from build123d import *

# Parameters (mm, degrees)
F1_DEPTH     = 6.35
F2_T1_DEPTH  = 59.8574546933
F2_T3_DEPTH  = 28.1503971994
F2_T6_ANGLE  = 90
F2_T8_ANGLE  = 90
F2_T10_ANGLE = 90
F2_T12_ANGLE = 90


# Not quite as in the source:
# - a fillet or chamfer that OpenCascade refuses, or shapes differently, is made with other operations: its cross-section is extruded or revolved along the edge and cut away or added


with BuildPart() as f1:
    # F0 (on Top) → F1 (new body)
    with BuildSketch(Plane.XY):
        with BuildLine():
            Line((20.4174276441, 0), (-20.4329695553, 0))
            Line((-20.4329695553, 0), (-20.4329695553, -47.1574546933))
            ThreePointArc((-20.4329695553, -47.1574546933), (-18.5730976158, -51.6475827539), (-14.0829695553, -53.5074546933))
            Line((-14.0829695553, -53.5074546933), (14.0674276441, -53.5074546933))
            ThreePointArc((14.0674276441, -53.5074546933), (18.5575557047, -51.6475827539), (20.4174276441, -47.1574546933))
            Line((20.4174276441, -47.1574546933), (20.4174276441, 0))
        make_face()
    extrude(amount=F1_DEPTH)

    # F2: fillet of radius 5.08 on 10 edges, made by hand

    # F2_s2 → F2_t1 (cut)
    with BuildSketch(Plane.XZ.offset(-12.7)):
        with BuildLine():
            ThreePointArc((20.4174276441, 1.27), (18.9295300926, 4.8621024484), (15.3374276441, 6.35))
            Line((15.3374276441, 6.35), (20.4174276441, 6.35))
            Line((20.4174276441, 6.35), (20.4174276441, 1.27))
        make_face()
        with BuildLine():
            ThreePointArc((20.4174276441, 5.08), (18.9295300926, 1.4878975516), (15.3374276441, 0))
            Line((15.3374276441, 0), (20.4174276441, 0))
            Line((20.4174276441, 0), (20.4174276441, 5.08))
        make_face()
        with BuildLine():
            ThreePointArc((-20.4329695553, 1.27), (-18.9450720037, 4.8621024484), (-15.3529695553, 6.35))
            Line((-15.3529695553, 6.35), (-20.4329695553, 6.35))
            Line((-20.4329695553, 6.35), (-20.4329695553, 1.27))
        make_face()
        with BuildLine():
            ThreePointArc((-20.4329695553, 5.08), (-18.9450720037, 1.4878975516), (-15.3529695553, 0))
            Line((-15.3529695553, 0), (-20.4329695553, 0))
            Line((-20.4329695553, 0), (-20.4329695553, 5.08))
        make_face()
    extrude(amount=F2_T1_DEPTH, mode=Mode.SUBTRACT)

    # F2_s4 → F2_t3 (cut)
    with BuildSketch(Plane.YZ.offset(-14.0829695553)):
        with BuildLine():
            ThreePointArc((-53.5074546933, 5.08), (-52.0195571417, 1.4878975516), (-48.4274546933, 0))
            Line((-48.4274546933, 0), (-53.5074546933, 0))
            Line((-53.5074546933, 0), (-53.5074546933, 5.08))
        make_face()
        with BuildLine():
            ThreePointArc((-53.5074546933, 1.27), (-52.0195571417, 4.8621024484), (-48.4274546933, 6.35))
            Line((-48.4274546933, 6.35), (-53.5074546933, 6.35))
            Line((-53.5074546933, 6.35), (-53.5074546933, 1.27))
        make_face()
    extrude(amount=F2_T3_DEPTH, mode=Mode.SUBTRACT)

    # F2_s5 → F2_t6 (revolve, cut)
    with BuildSketch(Plane.YZ.offset(14.0674276441)):
        with BuildLine():
            ThreePointArc((-53.5074546933, 1.27), (-52.0195571417, 4.8621024484), (-48.4274546933, 6.35))
            Line((-48.4274546933, 6.35), (-53.5074546933, 6.35))
            Line((-53.5074546933, 6.35), (-53.5074546933, 1.27))
        make_face()
    revolve(axis=Axis((14.0674276441, -47.1574546933, 6.35), (0, 0, 1)), revolution_arc=F2_T6_ANGLE, mode=Mode.SUBTRACT)

    # F2_s7 → F2_t8 (revolve, cut)
    with BuildSketch(Plane.YZ.offset(14.0674276441)):
        with BuildLine():
            ThreePointArc((-53.5074546933, 5.08), (-52.0195571417, 1.4878975516), (-48.4274546933, 0))
            Line((-48.4274546933, 0), (-53.5074546933, 0))
            Line((-53.5074546933, 0), (-53.5074546933, 5.08))
        make_face()
    revolve(axis=Axis((14.0674276441, -47.1574546933, 0), (0, 0, 1)), revolution_arc=F2_T8_ANGLE, mode=Mode.SUBTRACT)

    # F2_s9 → F2_t10 (revolve, cut)
    with BuildSketch(Plane.XZ.offset(47.1574546933)):
        with BuildLine():
            ThreePointArc((-20.4329695553, 1.27), (-18.9450720037, 4.8621024484), (-15.3529695553, 6.35))
            Line((-15.3529695553, 6.35), (-20.4329695553, 6.35))
            Line((-20.4329695553, 6.35), (-20.4329695553, 1.27))
        make_face()
    revolve(axis=Axis((-14.0829695553, -47.1574546933, 6.35), (0, 0, 1)), revolution_arc=F2_T10_ANGLE, mode=Mode.SUBTRACT)

    # F2_s11 → F2_t12 (revolve, cut)
    with BuildSketch(Plane.XZ.offset(47.1574546933)):
        with BuildLine():
            ThreePointArc((-20.4329695553, 5.08), (-18.9450720037, 1.4878975516), (-15.3529695553, 0))
            Line((-15.3529695553, 0), (-20.4329695553, 0))
            Line((-20.4329695553, 0), (-20.4329695553, 5.08))
        make_face()
    revolve(axis=Axis((-14.0829695553, -47.1574546933, 0), (0, 0, 1)), revolution_arc=F2_T12_ANGLE, mode=Mode.SUBTRACT)


solid = f1.part
Build history of the part. All positions in model axes, mm. Give positions to 0.01 mm unless a question says otherwise; leave off trailing zeros. Order: outer loops, then holes, each group sorted by start corner. A loop starts at its lowest first (then second) coordinate and runs counter-clockwise, first axis right, second up. Notation, with made-up numbers: M 72,74 L 120,74 A32 ccw 120,108 Z; hole C 51.25,25.25 d7. An arc over 180 degrees is marked long. Put each result on its own line as item: value.
Item 1: Cut at B-B on x = -10. Write the cut outline in (y, z) (3 decimals).
Results are:
outline: M -53.137,3.175 A5.08 ccw -48.427,0 L 0,0 L 0,6.35 L -48.427,6.35 A5.08 ccw Z
Item 2: Drop a flat-ended pin along its axis: pin 1 Ø1 at (y, z) = (-33.5, 1) entering from +X. Give the stop position or say it passes through.
Results are:
pin 1: x = 18.94
Item 3: Cut at A-A on y = -12. Write the cut outline in (x, z) (3 decimals), then the cut area to 3 significant figures.
Results are:
outline: M -20.062,3.175 A5.08 ccw -15.353,0 L 15.337,0 A5.08 ccw 20.047,3.175 A5.08 ccw 15.337,6.35 L -15.353,6.35 A5.08 ccw Z
area: 238 mm2
Item 4: Wall check: probe 1 along X at (y, z) = (-46, 0.5); probe 2 along Y at (x, z) = (13.5, 2.5); probe 3 along X at (y, z) = (-8, 1.25). Give the ranges that are in metal, low to high.
Results are:
probe 1: -17.55 to 17.54
probe 2: -52.8 to 0
probe 3: -18.69 to 18.67
